Can you work these out from the model? Positions are in its coordinate system, mm. Face numbers are marked on the shaded views. A direction names the side the tool comes from. Give positions to 0.01 mm unless a question says otherwise; leave off trailing zeros. Write each loop counter-clockwise with the first axis right and the second up, starting at its lowest first coordinate (ties: lowest second). Pieces come first, ordered by that corner, then holes. Notation, with made-up numbers: M 32,-31.5 L 91,-31.5 A27 cw 91,-15.5 Z; hole C -1.75,5 d10. An arc over 180 degrees is marked long. Use CSV: the item, a comma, the result in double quotes. Start each with the question number.
from build123d import *

# Parameters (mm, degrees)
F0_W           = 15
F0_H           = 30
F1_DEPTH       = 5
F3_D           = 5
F3_CSINK_D     = 11.2
F3_CSINK_ANGLE = 90
F4_W           = 15
F4_H           = 4
F5_DEPTH       = 8.5
F6_W           = 15
F6_H           = 1.9
F7_DEPTH       = 3
F8_R           = 1


with BuildPart() as f1:
    # F0 (on Front) → F1 (new body)
    with BuildSketch(Plane.XZ):
        Rectangle(F0_W, F0_H)
    extrude(amount=F1_DEPTH)

    # F3 (through all)
    with Locations(Plane.XZ.offset(5)):
        with Locations((0, 7)):
            CounterSinkHole(F3_D / 2, F3_CSINK_D / 2, counter_sink_angle=F3_CSINK_ANGLE)

    # F4 (on face) → F5 (join)
    with BuildSketch(Plane.XZ.offset(5)):
        with Locations((0, -13)):
            Rectangle(F4_W, F4_H)
    extrude(amount=F5_DEPTH)

    # F6 (on face) → F7 (join)
    with BuildSketch(Plane.XY.offset(-11)):
        with Locations((0, -12.55)):
            Rectangle(F6_W, F6_H)
    extrude(amount=F7_DEPTH)

    # F8
    f8_edges = [f1.edges().sort_by_distance(p)[0] for p in [
        (0, -13.5, -8),
        (7.5, -13.5, -11.5),
        (-7.5, -13.5, -11.5),
        (0, -13.5, -15),
        (7.5, -6.75, -15),
        (-7.5, -6.75, -15),
    ]]
    fillet(f8_edges, radius=F8_R)


solid = f1.part
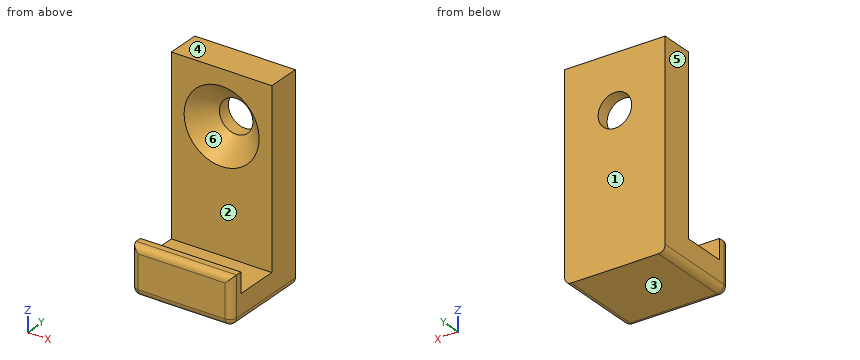
(1) Which directions (+Z, -Z, +X, -X, +Y, -Y) give clear straight access to the entire face, cutting with the end or side of a thin tool? Please do the marked faces 1 and 2.
(2) I want a section at C-C (y = -4). Write out the boundary of the cut face in (x, z), and give its area (3 significant figures).
(3) I want a section at B-B (z = 7). Write out the boundary of the cut face in (x, y), and give its area (3 significant figures).
(4) Thinking about a two-plate mould opening in Z: for the marked faces 3, 4, 5 and 6, which applies, released by +Z, released by -Z, zero draft, split by the parting line, or undercut?
(5) I want a section at A-A (x = 0). Write out the boundary of the cut face in (y, z).
(6) Please list where these lines run through material, in increasing order: L1, parallel to Z at x = 0, y = -0.55; L2, parallel to X at y = -0.7, z = 7; L3, parallel to Z at x = 6.5, y = -11.75. Write a range as [from, to].
(7) I want a section at D-D (x = 6). Write out the boundary of the cut face in (y, z), and give its area (3 significant figures).
(8) Will this pin go through, and if not, where does the flat tip stop? pin 1 Ø1 at (x, y) = (3, -12) entering from +Z.
Geometry results:
1,face 1,"+Z, -Z, +X, -X, +Y"
1,face 2,"+Z, +X, -X"
2,outline,"M -7.5,-14 A1 ccw -6.5,-15 L 6.5,-15 A1 ccw 7.5,-14 L 7.5,15 L -7.5,15 Z; hole C 0,7 d9.2"
2,area,"383 mm2"
3,outline,"M -7.5,-5 L -5.6,-5 L -2.5,-1.9 L -2.5,0 L -7.5,0 Z; M 2.5,-1.9 L 5.6,-5 L 7.5,-5 L 7.5,0 L 2.5,0 Z"
3,area,"40.4 mm2"
4,face 3,"released by -Z"
4,face 4,"released by +Z"
4,face 5,"zero draft"
4,face 6,"undercut"
5,outline,"M -13.5,-14 A1 ccw -12.5,-15 L 0,-15 L 0,4.5 L -1.9,4.5 L -5,1.4 L -5,-11 L -11.6,-11 L -11.6,-8 L -12.5,-8 A1 ccw -13.5,-9 Z; M -5,12.6 L -1.9,9.5 L 0,9.5 L 0,15 L -5,15 Z"
6,L1,"z = [-15, 4.5], [9.5, 15]"
6,L2,"x = [-7.5, -2.5], [2.5, 7.5]"
6,L3,"z = [-15, -8]"
7,outline,"M -13.5,-14 A1 ccw -12.5,-15 L 0,-15 L 0,15 L -5,15 L -5,-11 L -11.6,-11 L -11.6,-8 L -12.5,-8 A1 ccw -13.5,-9 Z"
7,area,"189 mm2"
8,pin 1,"stops at z = -8"
